The drawing under review shows one solid part. Ordinate dimensions are in mm from its lowest x, y, z. A direction names the side the tool comes from. Round coordinates to 2 decimals unless told otherwise and drop trailing zeros. Order: outer loops, then holes, each group sorted by start corner. A loop starts at its lowest first (then second) coordinate and runs counter-clockwise, first axis right, second up. Notation, with made-up numbers: M -17,45.5 L 1,45.5 A9 cw 1,52.5 Z; hole C 69.5,40 d6. An arc over 180 degrees is marked long. Answer as a JSON object with one key per item and string values. Group by question number.
1. Add section B-B on z = 15. State the section outline as (x, y) points, and give its area (3 significant figures).
2. Mouldability with a two-part tool opening along X and no side actions: class the marked faces 1, 2 and 3 as released by +X, released by -X, zero draft, split by the parting line, or undercut.
3. To check wall thickness, follow probe 1 along Z at (x, y) = (123, 11.5); probe 2 along X at (y, z) = (41, 26); probe 3 along Y at (x, z) = (102, 6). State the ranges of each line that lie inside material, in increasing order. Write a range as [from, to].
4. Add section C-C on y = 24. State the section outline as (x, z) points, and give its area (3 significant figures).
5. Add section A-A on x = 132. State the section outline as (y, z) points.
6. Machinability: for the marked faces 4 and 5, which of the approach directions +Z, -Z, +X, -X, +Y, -Y give a long, thin tool a straight path to every point of the face, cutting with its end or side? Answer none if there is none.
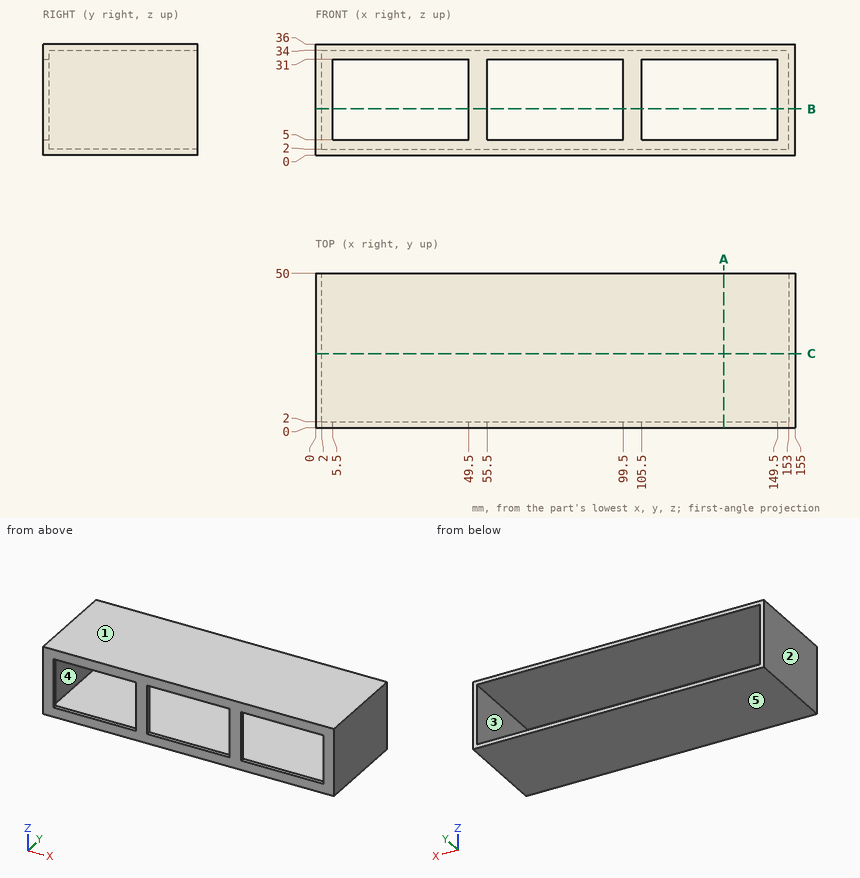
Recorded:
{
 "1": {"outline": "M 0,0 L 5.5,0 L 5.5,2 L 2,2 L 2,50 L 0,50 Z; M 49.5,0 L 55.5,0 L 55.5,2 L 49.5,2 Z; M 99.5,0 L 105.5,0 L 105.5,2 L 99.5,2 Z; M 149.5,0 L 155,0 L 155,50 L 153,50 L 153,2 L 149.5,2 Z", "area": "238 mm²"},
 "2": {"face 1": "zero draft", "face 2": "released by -X", "face 3": "undercut"},
 "3": {"probe 1": "z = [0, 2], [34, 36]", "probe 2": "x = [0, 2], [153, 155]", "probe 3": "y = [0, 2]"},
 "4": {"outline": "M 0,0 L 155,0 L 155,36 L 0,36 Z; hole M 2,2 L 153,2 L 153,34 L 2,34 Z", "area": "748 mm²"},
 "5": {"outline": "M 0,0 L 50,0 L 50,2 L 2,2 L 2,5 L 0,5 Z; M 0,31 L 2,31 L 2,34 L 50,34 L 50,36 L 0,36 Z"},
 "6": {"face 4": "+Y", "face 5": "-Z, +X, -X, +Y, -Y"}
}
